Model file for the job. Use its own axes, mm. Face numbers are marked on the shaded views. A direction names the side the tool comes from. Give positions to 0.01 mm unless a question says otherwise; leave off trailing zeros. Order: outer loops, then holes, each group sorted by start corner. A loop starts at its lowest first (then second) coordinate and runs counter-clockwise, first axis right, second up. Notation, with made-up numbers: (12, 42.5) -> (23, 42.5) arc R23 cw to (23, 59.5) -> close; hole circle Ø8 at (87, -11.5). An arc over 180 degrees is marked (long way). Answer in a Markdown table with one row per item. Add a question column.
from build123d import *

# Parameters (mm, degrees)
SKETCH1_W               = 50
SKETCH1_H               = 40
BOSS_EXTRUDE1_DEPTH     = 25
BOSS_EXTRUDE2_DEPTH     = 50
BOSS_EXTRUDE3_DEPTH     = 265
SKETCH4_W               = 10.5
SKETCH4_H               = 21
BOSS_EXTRUDE4_DEPTH     = 40
CUT_EXTRUDE3_DEPTH      = 388.585923019
CUT_EXTRUDE3_DEPTH_BACK = 25
SKETCH5_R               = 5


with BuildPart() as part:
    # Sketch1 → Boss-Extrude1 (new body)
    with BuildSketch(Plane(origin=(0, 0, 0), x_dir=(1, 0, 0), z_dir=(0, 1, 0))):
        with Locations((-89.035087719, 3.684210526)):
            Rectangle(SKETCH1_W, SKETCH1_H)
    extrude(amount=BOSS_EXTRUDE1_DEPTH)

    # Sketch2 → Boss-Extrude2 (add)
    with BuildSketch(Plane(origin=(0, 25, 0), x_dir=(1, 0, 0), z_dir=(0, 1, 0))):
        with BuildLine():
            ThreePointArc((-65.611981025, 3.684210526), (-71.223390651, 17.231351748), (-84.770531873, 22.842761374))
            Line((-84.770531873, 22.842761374), (-84.770531873, -15.474340321))
            ThreePointArc((-84.770531873, -15.474340321), (-71.223390651, -9.862930696), (-65.611981025, 3.684210526))
        make_face()
        with BuildLine():
            Line((-84.770531873, -15.474340321), (-84.770531873, 22.842761374))
            ThreePointArc((-84.770531873, 22.842761374), (-103.929082721, 3.684210526), (-84.770531873, -15.474340321))
        make_face()
    extrude(amount=BOSS_EXTRUDE2_DEPTH)

    # Sketch3 → Boss-Extrude3 (add)
    with BuildSketch(Plane.ZY.offset(114.035087719)):
        with BuildLine():
            Line((-3.684210526, 22.014273548), (-3.684210526, 24.28635832))
            ThreePointArc((-3.684210526, 24.28635832), (-15.470568846, 12.5), (-3.684210526, 0.71364168))
            Line((-3.684210526, 0.71364168), (-3.684210526, 2.985726452))
            ThreePointArc((-3.684210526, 2.985726452), (-13.198484074, 12.5), (-3.684210526, 22.014273548))
        make_face()
        with BuildLine():
            ThreePointArc((7.349913455, 16.643229465), (3.027147584, 22.188958394), (-3.684210526, 24.28635832))
            Line((-3.684210526, 24.28635832), (-3.684210526, 22.014273548))
            ThreePointArc((-3.684210526, 22.014273548), (3.043396817, 19.227607344), (5.830063022, 12.5))
            Line((5.830063022, 12.5), (5.830063022, 16.643229465))
            Line((5.830063022, 16.643229465), (7.349913455, 16.643229465))
        make_face()
        with BuildLine():
            ThreePointArc((8.102147793, 12.5), (7.912564487, 14.605481352), (7.349913455, 16.643229465))
            Line((7.349913455, 16.643229465), (5.830063022, 16.643229465))
            Line((5.830063022, 16.643229465), (5.830063022, 12.5))
            Line((5.830063022, 12.5), (5.830063022, 8.73562524))
            Line((5.830063022, 8.73562524), (7.484841587, 8.73562524))
            ThreePointArc((7.484841587, 8.73562524), (7.946797442, 10.592673056), (8.102147793, 12.5))
        make_face()
        with BuildLine():
            Line((-3.684210526, 2.985726452), (-3.684210526, 0.71364168))
            ThreePointArc((-3.684210526, 0.71364168), (3.191470264, 2.926951577), (7.484841587, 8.73562524))
            Line((7.484841587, 8.73562524), (5.830063022, 8.73562524))
            Line((5.830063022, 8.73562524), (5.830063022, 12.5))
            ThreePointArc((5.830063022, 12.5), (3.043396817, 5.772392656), (-3.684210526, 2.985726452))
        make_face()
        with BuildLine():
            Line((11.445254796, 16.643229465), (7.349913455, 16.643229465))
            ThreePointArc((7.349913455, 16.643229465), (7.912564487, 14.605481352), (8.102147793, 12.5))
            ThreePointArc((8.102147793, 12.5), (7.946797442, 10.592673056), (7.484841587, 8.73562524))
            Line((7.484841587, 8.73562524), (11.445254796, 8.73562524))
            Line((11.445254796, 8.73562524), (11.445254796, 16.643229465))
        make_face()
    extrude(amount=BOSS_EXTRUDE3_DEPTH)

    # Sketch4 → Boss-Extrude4 (add)
    with BuildSketch(Plane(origin=(-64.035087719, 0, 0), x_dir=(0, 0, -1), z_dir=(1, 0, 0))):
        with Locations((-1.565789474, 12.5)):
            Rectangle(SKETCH4_W, SKETCH4_H)
        with Locations((8.934210526, 12.5)):
            Rectangle(SKETCH4_W, SKETCH4_H)
    extrude(amount=BOSS_EXTRUDE4_DEPTH)

    # Sketch5 → Cut-Extrude3 (cut, two sides: drawn at the far end of the back side and taken through both)
    with BuildSketch(Plane.XY.offset(6.815789474).offset(-CUT_EXTRUDE3_DEPTH_BACK)):
        with BuildLine():
            Line((-24.035087719, 23), (-34.535087719, 23))
            ThreePointArc((-34.535087719, 23), (-27.110466517, 19.924621202), (-24.035087719, 12.5))
            Line((-24.035087719, 12.5), (-24.035087719, 23))
        make_face()
        with BuildLine():
            Line((-24.035087719, 2), (-24.035087719, 12.5))
            ThreePointArc((-24.035087719, 12.5), (-27.110466517, 5.075378798), (-34.535087719, 2))
            Line((-34.535087719, 2), (-24.035087719, 2))
        make_face()
        with Locations(Location((-34.535087719, 12.5, 0), (0, 0, 90))):
            Circle(SKETCH5_R)
    extrude(amount=CUT_EXTRUDE3_DEPTH + CUT_EXTRUDE3_DEPTH_BACK, mode=Mode.SUBTRACT)


solid = part.part
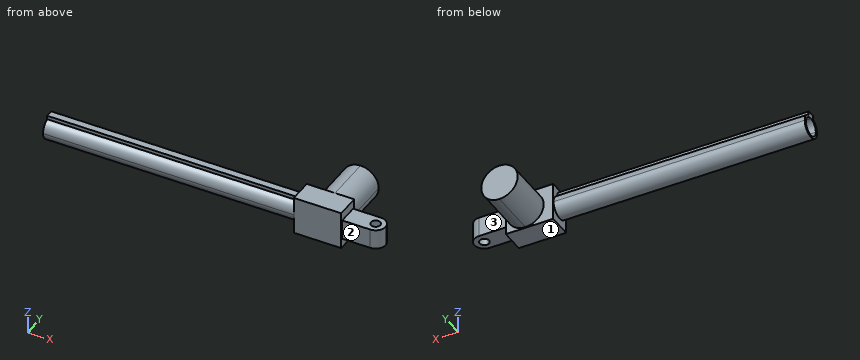
Item 1: Wall check: line 1 (Y direction, x = -171, z = -4); line 2 (Z direction, x = -180, y = 13); line 3 (X direction, y = 12, z = -9). Give the ranges that are in metal, low to high.
Item 2: Which spindle directions (+Z, -Z, +X, -X, +Y, -Y) get a long thin tool onto all of the face, cutting with end or side? Do the marked faces 1, 2 and 3. Say none if no direction does.
Item 3: Saw through at D-D on x = -92. List the corners of the cut face in (y, z), plus the area to 3 significant figures.
Item 4: Saw through at A-A on x = -278. List the corners of the cut face in (y, z).
Item 5: Saw through at B-B on z = 0. List the corners of the cut face in (x, y).
Item 6: Saw through at C-C on y = 66. List the corners of the cut face in (x, z), plus the area to 3 significant figures.
Item 7: Pin check, flat tips, straight feed: pin 1 Ø2 at (x, z) = (-190, 9.5) entering from +Y; pin 2 Ø16 at (x, y) = (-34.54, 12.5) entering from -Z; pin 3 Ø3 at (y, z) = (53, -11) entering from +X; pin 4 Ø12 at (x, y) = (-208, 35) entering from +Z. Stop position of each tip, or through.
Evaluation:
| question | item | result |
|---|---|---|
| 1 | line 1 | y = 0.72 to 2.99, 22.01 to 24.28 |
| 1 | line 2 | z = -15.46 to -13.19, 5.82 to 11.45 |
| 1 | line 3 | x = -114.04 to -39.51, -29.56 to -24.05 |
| 2 | face 1 | -Z, +X, -X, +Y, -Y |
| 2 | face 2 | +Z, -Z, +X, -Y |
| 2 | face 3 | +Z, -Z, +X, +Y |
| 3 | outline | (0, -23.68) -> (25, -23.68) -> (25, -21.43) -> (75, -21.43) -> (75, 14.06) -> (25, 14.06) -> (25, 16.32) -> (0, 16.32) -> close |
| 3 | area | 2,770 mm2 |
| 4 | outline | (8.74, 7.48) arc R11.79 ccw (long way) to (16.64, 7.35) -> (16.64, 11.45) -> (8.74, 11.45) -> close; hole circle Ø19.03 at (12.5, -3.68) |
| 5 | outline | (-379.04, 1.3) -> (-114.04, 1.3) -> (-114.04, 0) -> (-64.04, 0) -> (-64.04, 2) -> (-34.54, 2) arc R10.5 ccw to (-34.54, 23) -> (-64.04, 23) -> (-64.04, 25) -> (-65.97, 25) -> (-65.97, 75) -> (-103.57, 75) -> (-103.57, 25) -> (-114.04, 25) -> (-114.04, 23.7) -> (-379.04, 23.7) -> (-379.04, 21.27) -> (-114.04, 21.27) -> (-114.04, 3.73) -> (-379.04, 3.73) -> close; hole circle Ø10 at (-34.54, 12.5) |
| 6 | outline | circle Ø38.32 at (-84.77, -3.68) |
| 6 | area | 1,150 mm2 |
| 7 | pin 1 | stops at y = 16.64 |
| 7 | pin 2 | stops at z = -14.18 |
| 7 | pin 3 | stops at x = -66.52 |
| 7 | pin 4 | passes through |
